Verification items for the finished model (mm, model axes). A direction names the side the tool comes from. Round coordinates to 2 decimals unless told otherwise and drop trailing zeros. Write each loop counter-clockwise with the first axis right and the second up, starting at its lowest first coordinate (ties: lowest second). Pieces come first, ordered by that corner, then holes.
from build123d import *

# Parameters (mm, degrees)
SKETCH1_R                    = 25.4
SKETCH1_R_2                  = 23.01875
BOSS_EXTRUDE1_DEPTH          = 679.45
SKETCH2_R                    = 28.575
SKETCH2_R_2                  = 25.4
BOSS_EXTRUDE2_DEPTH          = 25.4
SKETCH4_R                    = 1.89865
CUT_EXTRUDE1_DEPTH           = 683.618175501
SKETCH5_R                    = 25.4
BOSS_EXTRUDE4_DEPTH          = 6.35
SKETCH6_R                    = 12.7
BOSS_EXTRUDE5_DEPTH          = 31.75
SKETCH7_R                    = 9.525
BOSS_EXTRUDE6_DEPTH          = 444.5
F_1_4_CLEARANCE_HOLE1_REACH  = 684.618
F_1_4_CLEARANCE_HOLE1_BORE_R = 3.3782


with BuildPart() as part:
    # Sketch1 → Boss-Extrude1 (new body)
    with BuildSketch(Plane(origin=(0, 0, 0), x_dir=(1, 0, 0), z_dir=(0, 1, 0))):
        with Locations(Location((0, 0, 0), (0, 0, 270))):
            Circle(SKETCH1_R)
        with Locations(Location((0, 0, 0), (0, 0, 270))):
            Circle(SKETCH1_R_2, mode=Mode.SUBTRACT)
    extrude(amount=BOSS_EXTRUDE1_DEPTH)

    # Sketch2 → Boss-Extrude2 (add)
    with BuildSketch(Plane(origin=(0, 0, 0), x_dir=(-1, 0, 0), z_dir=(0, -1, 0))):
        with Locations(Location((0, 0, 0), (0, 0, 90))):
            Circle(SKETCH2_R)
        with Locations(Location((0, 0, 0), (0, 0, 90))):
            Circle(SKETCH2_R_2, mode=Mode.SUBTRACT)
    extrude(amount=-BOSS_EXTRUDE2_DEPTH)

    # Sketch4 → Cut-Extrude1 (cut, through all)
    with BuildSketch(Plane(origin=(15.595341272, 0, -20.048574278), x_dir=(-0.7893139479687464, 0, -0.6139898138747834), z_dir=(0.6139898138747834, 0, -0.7893139479687464))):
        with Locations((0, 55.5625)):
            Circle(SKETCH4_R)
        with Locations((0, 42.8625)):
            Circle(SKETCH4_R)
        with Locations((0, 30.1625)):
            Circle(SKETCH4_R)
    extrude(amount=-CUT_EXTRUDE1_DEPTH, mode=Mode.SUBTRACT)

    # Sketch5 → Boss-Extrude4 (add)
    with BuildSketch(Plane.XZ):
        with Locations(Location((0, 0, 0), (0, 0, 270))):
            Circle(SKETCH5_R)
    extrude(amount=BOSS_EXTRUDE4_DEPTH)

    # Sketch6 → Boss-Extrude5 (add)
    with BuildSketch(Plane.XZ.offset(6.35)):
        with Locations(Location((0, 0, 0), (0, 0, 270))):
            Circle(SKETCH6_R)
    extrude(amount=BOSS_EXTRUDE5_DEPTH)

    # Sketch7 → Boss-Extrude6 (add)
    with BuildSketch(Plane.XZ.offset(38.1)):
        with Locations(Location((0, 0, 0), (0, 0, 270))):
            Circle(SKETCH7_R)
    extrude(amount=BOSS_EXTRUDE6_DEPTH)

    # 1/4 Clearance Hole1 bore → 1/4 Clearance Hole1 (cut, up to next)
    with BuildSketch(Plane(origin=(20.048574278, 0, 15.595341272), x_dir=(0.6139898138747835, 0, -0.7893139479687464), z_dir=(0.7893139479687464, 0, 0.6139898138747835)), mode=Mode.PRIVATE) as f_1_4_clearance_hole1_sk1:
        with Locations((0, 666.75)):
            Circle(F_1_4_CLEARANCE_HOLE1_BORE_R)
    f_1_4_clearance_hole1_tool1 = extrude(f_1_4_clearance_hole1_sk1.sketch, amount=-F_1_4_CLEARANCE_HOLE1_REACH, mode=Mode.PRIVATE) & part.part
    add(f_1_4_clearance_hole1_tool1.solids().sort_by_distance((20.048574, 666.75, 15.595341))[0], mode=Mode.SUBTRACT)


solid = part.part
Q1. Sectioned sample at A-A (x = 0). Enter the section's corners in (y, z) (3 decimals), plus the area to 3 significant figures.
Recorded:
outline: (-482.6, -9.525) - (-38.1, -9.525) - (-38.1, -12.7) - (-6.35, -12.7) - (-6.35, -25.4) - (0, -25.4) - (0, -28.575) - (25.4, -28.575) - (25.4, -25.4) - (679.45, -25.4) - (679.45, -23.019) - (0, -23.019) - (0, 23.019) - (679.45, 23.019) - (679.45, 25.4) - (25.4, 25.4) - (25.4, 28.575) - (0, 28.575) - (0, 25.4) - (-6.35, 25.4) - (-6.35, 12.7) - (-38.1, 12.7) - (-38.1, 9.525) - (-482.6, 9.525) - close
area: 13,000 mm2
Q2. Sectioned sample at C-C (y = -236). Enter the section's corners in (x, z) (3 decimals).
Recorded:
outline: circle Ø19.05 at (0, 0)
Q3. Sectioned sample at D-D (y = 443). Enter the section's corners in (x, z).
Recorded:
outline: circle Ø50.8 at (0, 0); hole circle Ø46.04 at (0, 0)
Q4. Release check for a two-part mould opening along X. For faces 4 (the flat face through (0, -482.6, 0)), 5 (the cylindrical face through (-15.456, -3.131, 20.157)), 6 (the cylindrical face through (-22.47, 334.97, -4.99)) record: released by +X, released by -X, zero draft, split by the parting line, or undercut.
Recorded:
face 4: zero draft
face 5: split by the parting line
face 6: undercut
Q5. Material ranges on line 1 along X through (y, z) = (496, 0); line 2 along Y through (x, z) = (4, -11.5); line 3 along Y through (x, z) = (10, 15.5), recorded low to high.
Recorded:
line 1: x = -25.4 to -23.02, 23.02 to 25.4
line 2: y = -38.1 to 0
line 3: y = -6.35 to 0
Q6. Depth check by flat-ended pin: P1, Ø8, axis at y = 522, z = 13.5, coming from the -X side; P2, Ø12, axis at y = 212.5, z = -2.5, coming from the +X side; P3, Ø3, axis at x = -5, y = 186, coming from the +Z side. Enter the tip coordinate at first touch or a pass-through.
Recorded:
P1: stops at x = -23.56
P2: stops at x = 25.4
P3: stops at z = 25.16
Q7. Tool access check on faces 1 (the cylindrical face through (1.256, 12.522, 28.547)), 2 (the cylindrical face through (-5.796, -257.238, 7.559)), 3 (the cylindrical face through (-15.456, 347.847, -20.157)). Record the directions out of +Z, -Z, +X, -X, +Y, -Y that give a thin tool (end or side, any length) a straight path to the whole face; none if there is none.
Recorded:
face 1: +Y, -Y
face 2: -Y
face 3: +Y
Q8. Sectioned sample at B-B (z = 0). Enter the section's corners in (x, y) (3 decimals), plus the area to 3 significant figures.
Recorded:
outline: (-28.575, 0) - (-25.4, 0) - (-25.4, -6.35) - (-12.7, -6.35) - (-12.7, -38.1) - (-9.525, -38.1) - (-9.525, -482.6) - (9.525, -482.6) - (9.525, -38.1) - (12.7, -38.1) - (12.7, -6.35) - (25.4, -6.35) - (25.4, 0) - (28.575, 0) - (28.575, 25.4) - (25.4, 25.4) - (25.4, 679.45) - (23.019, 679.45) - (23.019, 0) - (-23.019, 0) - (-23.019, 679.45) - (-25.4, 679.45) - (-25.4, 25.4) - (-28.575, 25.4) - close
area: 13,000 mm2
